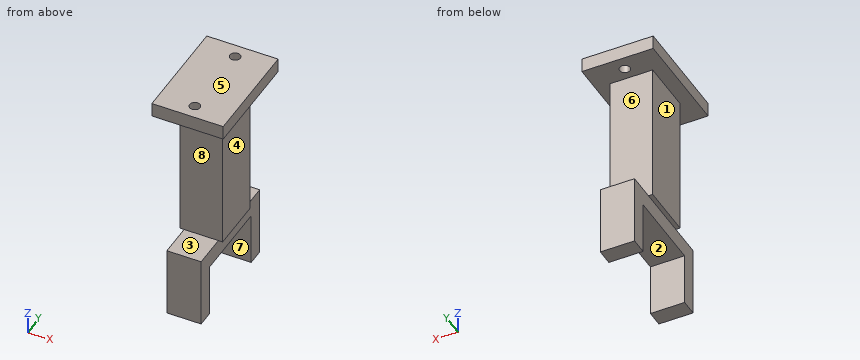
from build123d import *

# Parameters (mm, degrees)
SKETCH_1_W          = 20
SKETCH_1_H          = 30
SKETCH_1_R          = 1.45
EXTRUDE_1_DEPTH     = 4
SKETCH_2_W          = 12
SKETCH_2_H          = 15
EXTRUDE_2_DEPTH     = 40
SKETCH_3_W          = 9.6
SKETCH_3_H          = 32
EXTRUDE_3_DEPTH     = 20
SKETCH_4_W          = 9.6
SKETCH_4_H          = 22.7
EXTRUDE_4_DEPTH     = 15
SKETCH_4_2_W        = 9.6
SKETCH_4_2_H        = 22.7
CUT_EXTRUDE_1_DEPTH = 15


with BuildPart() as part:
    # Эскиз1 → Бобышка-Вытянуть1 (new body)
    with BuildSketch(Plane.XY):
        with Locations((-1.805054152, 0.992779783)):
            Rectangle(SKETCH_1_W, SKETCH_1_H)
        with Locations((-1.805054152, 11.992779783)):
            Circle(SKETCH_1_R, mode=Mode.SUBTRACT)
        with Locations((-1.805054152, -10.007220217)):
            Circle(SKETCH_1_R, mode=Mode.SUBTRACT)
    extrude(amount=EXTRUDE_1_DEPTH)

    # Эскиз2 → Бобышка-Вытянуть2 (add)
    with BuildSketch(Plane(origin=(0, 0, 0), x_dir=(-1, 0, 0), z_dir=(0, 0, -1))):
        with Locations((1.805054152, 0.992779783)):
            Rectangle(SKETCH_2_W, SKETCH_2_H)
    extrude(amount=EXTRUDE_2_DEPTH)

    # Эскиз3 → Бобышка-Вытянуть3 (add)
    with BuildSketch(Plane(origin=(0, 0, -40), x_dir=(-1, 0, 0), z_dir=(0, 0, -1))):
        with Locations((1.805054152, 0.05753703)):
            Rectangle(SKETCH_3_W, SKETCH_3_H)
    extrude(amount=EXTRUDE_3_DEPTH)

    # Эскиз4 → Бобышка-Вытянуть4 (add)
    with BuildSketch(Plane(origin=(0, 0, -60), x_dir=(-1, 0, 0), z_dir=(0, 0, -1))):
        with Locations((1.805054152, 0.05753703)):
            Rectangle(SKETCH_4_W, SKETCH_4_H)
    extrude(amount=-EXTRUDE_4_DEPTH)

    # Эскиз4<2> → Вырез-Вытянуть1 (cut)
    with BuildSketch(Plane(origin=(0, 0, -60), x_dir=(-1, 0, 0), z_dir=(0, 0, -1))):
        with Locations((1.805054152, 0.05753703)):
            Rectangle(SKETCH_4_2_W, SKETCH_4_2_H)
    extrude(amount=-CUT_EXTRUDE_1_DEPTH, mode=Mode.SUBTRACT)


solid = part.part
Input: part model. Units: mm. Frame: model coordinates. Face numbers are marked on the shaded views. A direction names the side the tool comes from. Give positions to 0.01 mm unless a question says otherwise; leave off trailing zeros. Order: outer loops, then holes, each group sorted by start corner. A loop starts at its lowest first (then second) coordinate and runs counter-clockwise, first axis right, second up. Notation, with made-up numbers: (-24.5, 80) -> (13.5, 80) arc R18 cw to (13.5, 99) -> close; hole circle Ø2 at (-37, 22.25). An arc over 180 degrees is marked (long way). Use one line per item in the form item = value.
1) First-contact query: pin 1 Ø1 at (x, y) = (-7, 3.5) entering from -Z; pin 2 Ø16.5 at (y, z) = (3.5, -28.5) entering from -X; pin 3 Ø9.5 at (x, z) = (1, -12) entering from -Y. Flat tips, straight axial feed; report the tip coordinate or a pass-through.
Response values:
pin_1 = -45
pin_2 = -7.81
pin_3 = -6.51
2) Section C-C, the plane x = -2.5. Return loops of the section in (y, z), and give its area (3 significant figures).
Response values:
outline = (-15.94, -60) -> (-11.29, -60) -> (-11.29, -45) -> (11.41, -45) -> (11.41, -60) -> (16.06, -60) -> (16.06, -40) -> (8.49, -40) -> (8.49, 0) -> (10.72, 0) -> (10.72, 4) -> (-8.73, 4) -> (-8.73, 0) -> (-6.51, 0) -> (-6.51, -40) -> (-15.94, -40) -> close; (-14.01, 0) -> (-11.28, 0) -> (-11.28, 4) -> (-14.01, 4) -> close; (13.27, 0) -> (15.99, 0) -> (15.99, 4) -> (13.27, 4) -> close
area = 999 mm^2
3) Reachability of the marked faces 1, 2, 3 and 4 from +Z, -Z, +X, -X, +Y, -Y: full face, straight path, thin tool, end or side. Return the list, or none.
Response values:
face_1 = -Z, -X, +Y, -Y
face_2 = -Z, +X, -X
face_3 = +X, -X, -Y
face_4 = -Z, +X, +Y, -Y
4) Section D-D, the plane z = -18. Return loops of the section in (x, y), and give its area (3 significant figures).
Response values:
outline = (-7.81, -6.51) -> (4.19, -6.51) -> (4.19, 8.49) -> (-7.81, 8.49) -> close
area = 180 mm^2
5) Section B-B, the plane x = 1. Return loops of the section in (y, z), and give its area (3 significant figures).
Response values:
outline = (-15.94, -60) -> (-11.29, -60) -> (-11.29, -45) -> (11.41, -45) -> (11.41, -60) -> (16.06, -60) -> (16.06, -40) -> (8.49, -40) -> (8.49, 0) -> (15.99, 0) -> (15.99, 4) -> (-14.01, 4) -> (-14.01, 0) -> (-6.51, 0) -> (-6.51, -40) -> (-15.94, -40) -> close
area = 1,020 mm^2
6) Section A-A, the plane y = 5.5. Return loops of the section in (x, z), and give its area (3 significant figures).
Response values:
outline = (-11.81, 0) -> (-7.81, 0) -> (-7.81, -40) -> (-6.61, -40) -> (-6.61, -45) -> (2.99, -45) -> (2.99, -40) -> (4.19, -40) -> (4.19, 0) -> (8.19, 0) -> (8.19, 4) -> (-11.81, 4) -> close
area = 608 mm^2
7) Mould query, pull axis Y, two halves, no side actions, for the marked faces 5, 6, 7 and 8. Classes: pulls with the +Y half, pulls with the -Y half, needs draft (parallel to the pull), parting line crosses it, or undercut.
Response values:
face_5 = needs draft
face_6 = pulls with the +Y half
face_7 = undercut
face_8 = pulls with the -Y half
8) Line query: probe 1 along Z at (x, y) = (1, 13.5); probe 2 along Y at (x, z) = (-1.25, -53.5); probe 3 along Z at (x, y) = (-1.25, -7). Output: solid intervals per line, ascending.
Response values:
probe_1 = -60 to -40, 0 to 4
probe_2 = -15.94 to -11.29, 11.41 to 16.06
probe_3 = -45 to -40, 0 to 4
